```python
from build123d import *

# Parameters (mm, degrees)
F1_DEPTH = 1123.95
F2_W     = 122.435573
F2_H     = 50.8
F2_W_2   = 93.867282
F2_W_3   = 343.160421
F2_H_2   = 127
F3_DEPTH = 25.4
F4_R     = 0.79375
F5_DEPTH = 25.4
F6_R     = 4.7625
F7_DEPTH = 25.4


with BuildPart() as f1:
    # F0 (on Top) → F1 (new body)
    with BuildSketch(Plane.XY):
        Polygon((25.4, -9.525), (25.4, 9.525), (0, 9.525), (-7.890768, -9.525), align=None)
    extrude(amount=F1_DEPTH)

    # F2 (on Front) → F3 (cut)
    with BuildSketch(Plane.XZ):
        with Locations((22.446524, 25.4)):
            Rectangle(F2_W, F2_H)
        with Locations((2.720783, 755.65)):
            Rectangle(F2_W_2, F2_H)
        with Locations((-38.781822, 1060.45)):
            Rectangle(F2_W_3, F2_H_2)
    extrude(amount=F3_DEPTH, mode=Mode.SUBTRACT)

    # F4 (on Front) → F5 (cut)
    with BuildSketch(Plane.XZ):
        with Locations((12.7, 101.6)):
            Circle(F4_R)
        with Locations((12.7, 155.575)):
            Circle(F4_R)
        with Locations((12.7, 625.475)):
            Circle(F4_R)
        with Locations((12.7, 679.45)):
            Circle(F4_R)
        with Locations((-12.7, 625.475)):
            Circle(F4_R)
        with Locations((-12.7, 679.45)):
            Circle(F4_R)
        with Locations((-12.7, 101.6)):
            Circle(F4_R)
        with Locations((-12.7, 155.575)):
            Circle(F4_R)
    extrude(amount=-F5_DEPTH, mode=Mode.SUBTRACT)

    # F6 (on Front) → F7 (cut)
    with BuildSketch(Plane.XZ):
        with Locations((15.875, 254)):
            Circle(F6_R)
        with Locations((15.875, 482.6)):
            Circle(F6_R)
    extrude(amount=F7_DEPTH, mode=Mode.SUBTRACT)


solid = f1.part
```
Geometry: final body of the model. Coordinates: model frame, mm. A direction names the side the tool comes from. Coordinates: 2 decimals unless noted, no trailing zeros. Order: outer loops, then holes, each group sorted by start corner. A loop starts at its lowest first (then second) coordinate and runs counter-clockwise, first axis right, second up. Notation, with made-up numbers: (67, 83) - (95, 83) arc R20 cw to (95, 104) - close; hole circle Ø1 at (55.5, 3). An arc over 180 degrees is marked (long way). Write each question's results on one line, items separated by ' | '.
1) Pull-direction query (Z, two-part tool) for faces 4 (the flat face through (9, -9.525, 386)), 5 (the flat face through (11, 0, 756)); classes: pulls with the +Z half, pulls with the -Z half, needs draft (parallel to the pull), parting line crosses it, or undercut.
Results list:
face 4: needs draft | face 5: undercut
2) Section B-B, the plane z = 404. Return loops of the section in (x, y) (3 decimals).
Results list:
outline: (-7.891, -9.525) - (25.4, -9.525) - (25.4, 9.525) - (0, 9.525) - close
3) Section A-A, the plane y = -4. State how many separate pieces and enclosed holes the cut face has, plus the area to 3 significant figures.
Results list:
separate pieces: 2 | enclosed holes: 2 | area: 27,600 mm^2
4) Set-up query: faces 1 (the flat face through (25.4, 0, 554)), 2 (the flat face through (11, 0, 26)), 3 (the flat face through (11, 0, 1061)). Return all of +Z, -Z, +X, -X, +Y, -Y with unobstructed straight access to the full face (end or side cutting, diameter ignored); none if empty.
Results list:
face 1: +Z, -Z, +X, +Y, -Y | face 2: -Z, +X, -X, -Y | face 3: +Z, +X, -X, -Y
5) Pin query (flat end, axial travel): pin 1 (6 mm diameter, centred on y = -1.5, z = 322, fed in from -X); pin 2 (3 mm diameter, centred on x = 2.5, y = -3, fed in from -Z); pin 3 (7.5 mm diameter, centred on x = 15.875, z = 482.6, fed in from -Y). Return the tip coordinate at first contact, or that it passes through.
Results list:
pin 1: x = -5.81 | pin 2: z = 50.8 | pin 3: y = 0
6) Line query: line 1 (Z direction, x = 12.7, y = 2.5); line 2 (Z direction, x = 8.5, y = -7.75); line 3 (Z direction, x = 19, y = -5.75). Output: solid intervals per line, ascending. Write a range as from..to.
Results list:
line 1: 0..100.81, 102.39..154.78, 156.37..624.68, 626.27..678.66, 680.24..1123.95 | line 2: 50.8..730.25, 781.05..996.95 | line 3: 50.8..250.41, 257.59..479.01, 486.19..730.25, 781.05..996.95
